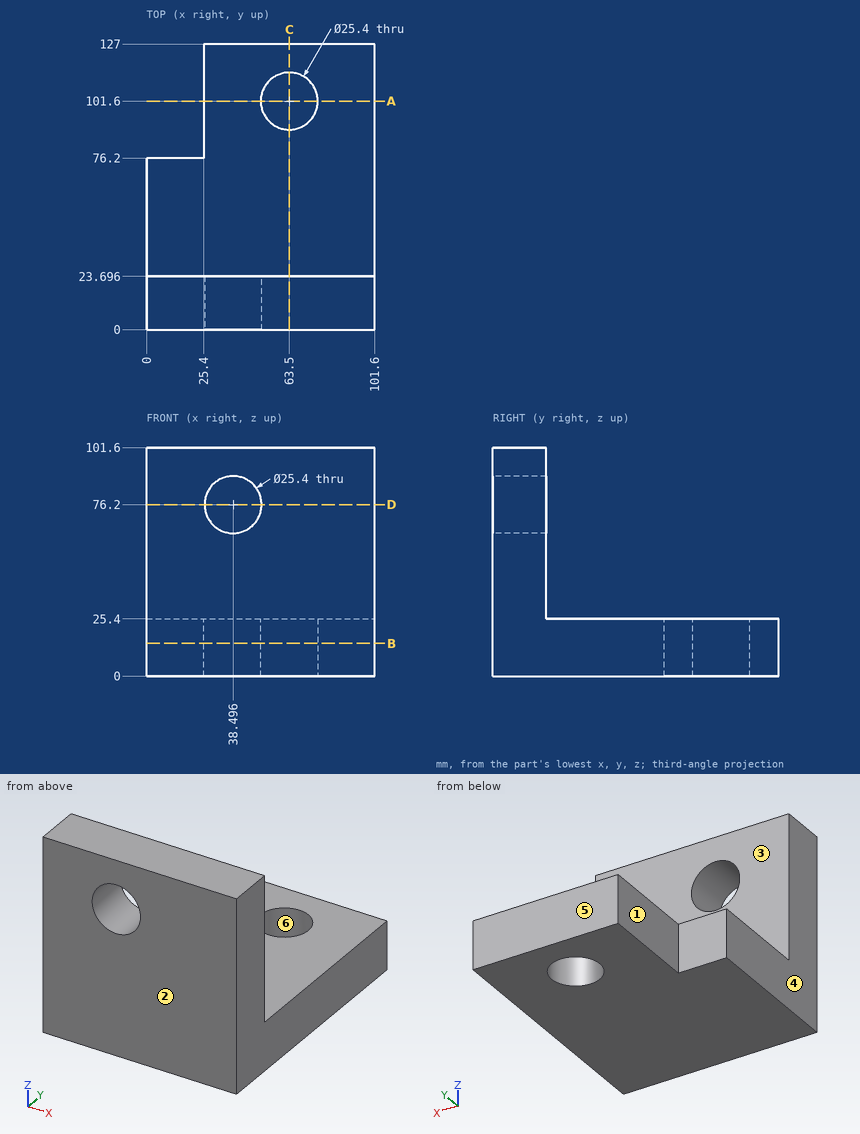
Part print with two shaded views. Sizes in mm from the minimum x, y, z corner. A direction names the side the tool comes from. Round coordinates to 2 decimals unless told otherwise and drop trailing zeros. Order: outer loops, then holes, each group sorted by start corner. A loop starts at its lowest first (then second) coordinate and runs counter-clockwise, first axis right, second up. Notation, with made-up numbers: (27, -11) -> (70, -11) arc R25 cw to (70, 24) -> close; hole circle Ø5 at (82, -2.5). An arc over 180 degrees is marked (long way). Use one line per item in the form item = value.
Item 1: Drill centre lines: line 1 (Y direction, x = 63, z = 16); line 2 (Z direction, x = 94.5, y = 103); line 3 (Y direction, x = 43.5, z = 32). Where is each one in solid material? Low to high.
Returned:
line_1 = 0 to 88.91, 114.29 to 127
line_2 = 0 to 25.4
line_3 = 0 to 23.7
Item 2: Cut at B-B, the plane z = 14.5. Write the cut outline in (x, y), and give its area (3 significant figures).
Returned:
outline = (0, 0) -> (101.6, 0) -> (101.6, 127) -> (25.4, 127) -> (25.4, 76.2) -> (0, 76.2) -> close; hole circle Ø25.4 at (63.5, 101.6)
area = 11,100 mm^2
Item 3: Cut at A-A, the plane y = 101.6. Write the cut outline in (x, z).
Returned:
outline = (25.4, 0) -> (50.8, 0) -> (50.8, 25.4) -> (25.4, 25.4) -> close; (76.2, 0) -> (101.6, 0) -> (101.6, 25.4) -> (76.2, 25.4) -> close
Item 4: Tool access for the marked faces 1, 2 and 3: list every direction of +Z, -Z, +X, -X, +Y, -Y with a clear straight run to the whole face (end or side of a thin tool).
Returned:
face_1 = +Z, -Z, -X, +Y
face_2 = +Z, -Z, +X, -X, -Y
face_3 = +Z, +X, -X, +Y
Item 5: Pull direction X, two halves, no side cores. Call the marked faces 4, 5 and 6: released by +X, released by -X, zero draft, split by the parting line, or undercut.
Returned:
face_4 = released by -X
face_5 = zero draft
face_6 = undercut
Item 6: Flat gauge pin, fed straight in: pin 1 Ø12.5 at (y, z) = (95, 11) entering from -X. Where does the tip first touch, or does it go through?
Returned:
pin_1 = 25.4
Item 7: Cut at C-C, the plane x = 63.5. Write the cut outline in (y, z), and give its area (3 significant figures).
Returned:
outline = (0, 0) -> (88.9, 0) -> (88.9, 25.4) -> (23.7, 25.4) -> (23.7, 101.6) -> (0, 101.6) -> close; (114.3, 0) -> (127, 0) -> (127, 25.4) -> (114.3, 25.4) -> close
area = 4,390 mm^2
Item 8: Cut at D-D, the plane z = 76.2. Write the cut outline in (x, y) (1 decimal).
Returned:
outline = (0, 0) -> (25.8, 0) -> (25.8, 23.7) -> (0, 23.7) -> close; (51.2, 0) -> (101.6, 0) -> (101.6, 23.7) -> (51.2, 23.7) -> close
